For this review, take the finished solid that the model builds, in its own axes (mm). Face numbers are marked on the shaded views. A direction names the side the tool comes from. Coordinates: 2 decimals unless noted, no trailing zeros. Write each loop counter-clockwise with the first axis right and the second up, starting at its lowest first coordinate (ties: lowest second). Pieces come first, ordered by that corner, then holes.
```python
from build123d import *

# Parameters (mm, degrees)
SKETCH1_R           = 17
SKETCH1_R_2         = 13
BOSS_EXTRUDE1_DEPTH = 10
SKETCH2_R           = 30
SKETCH2_R_2         = 13
BOSS_EXTRUDE2_DEPTH = 8
SKETCH6_R           = 17
SKETCH6_R_2         = 8.5
BOSS_EXTRUDE3_DEPTH = 3
SKETCH7_R           = 13
SKETCH7_R_2         = 9.5
BOSS_EXTRUDE4_DEPTH = 9
CUT_EXTRUDE2_START  = -1.8
SKETCH8_R           = 10
CUT_EXTRUDE2_DEPTH  = 1.2


with BuildPart() as part:
    # Sketch1 → Boss-Extrude1 (new body)
    with BuildSketch(Plane.XY):
        Circle(SKETCH1_R)
        Circle(SKETCH1_R_2, mode=Mode.SUBTRACT)
    extrude(amount=BOSS_EXTRUDE1_DEPTH)

    # Sketch2 → Boss-Extrude2 (add)
    with BuildSketch(Plane.XY.offset(10)):
        Circle(SKETCH2_R)
        Circle(SKETCH2_R_2, mode=Mode.SUBTRACT)
    extrude(amount=BOSS_EXTRUDE2_DEPTH)

    # Sketch6 → Boss-Extrude3 (add)
    with BuildSketch(Plane(origin=(0, 0, 0), x_dir=(-1, 0, 0), z_dir=(0, 0, -1))):
        with Locations(Location((0, 0, 0), (0, 0, 180))):
            Circle(SKETCH6_R)
        Circle(SKETCH6_R_2, mode=Mode.SUBTRACT)
    extrude(amount=-BOSS_EXTRUDE3_DEPTH)

    # Sketch7 → Boss-Extrude4 (add)
    with BuildSketch(Plane.XY.offset(3)):
        Circle(SKETCH7_R)
        Circle(SKETCH7_R_2, mode=Mode.SUBTRACT)
    extrude(amount=BOSS_EXTRUDE4_DEPTH)

    # Sketch8 → Cut-Extrude2 (cut)
    with BuildSketch(Plane.XY.offset(12).offset(CUT_EXTRUDE2_START)):
        Circle(SKETCH8_R)
    extrude(amount=-CUT_EXTRUDE2_DEPTH, mode=Mode.SUBTRACT)


solid = part.part
```
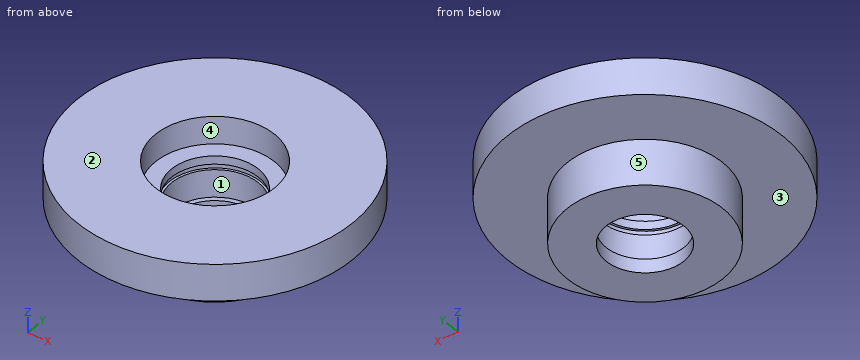
1) Consider section C-C (x = -11). Give the boundary of the cut face in (y, z), then the cut area to 3 significant figures.
2) The part is to be moulded in two halves that separate along Y. For the marked faces 3, 4 and 5, say which applies: pulls with the +Y half, pulls with the -Y half, needs draft (parallel to the pull), parting line crosses it, or undercut.
3) Clearance check with flat-ended pins moving along their axes: P1, Ø10, axis at y = 2, z = 13, coming from the +X side; P2, Ø6, axis at y = 13.5, z = 11.5, coming from the -X side; P3, Ø22, axis at x = 0, y = 0, coming from the +Z side; P4, Ø10, axis at y = -9.5, z = 14, coming from the +X side. State where each tip first meets the part, or that it passes through.
4) Consider section A-A (x = 0). Give the boundary of the cut face in (y, z), then the cut area to 3 significant figures.
5) For L1, parallel to Y at x = 0, z = 15.6; L2, parallel to Y at x = 0, z = 4.45; L3, parallel to Z at x = -24, y = 12, list the stretches that pass through material, from the lowest coordinate up.
6) Tool access review of the marked faces 1 and 2: name each direction out of +Z, -Z, +X, -X, +Y, -Y from which nothing blocks a thin tool from reaching the whole face with its end or side.
7) Consider section D-D (z = 2). Give the boundary of the cut face in (x, y).
Results:
1. outline: (-27.91, 10) - (-12.96, 10) - (-12.96, 0) - (12.96, 0) - (12.96, 10) - (27.91, 10) - (27.91, 18) - (6.93, 18) - (6.93, 12) - (-6.93, 12) - (-6.93, 18) - (-27.91, 18) - close
1. area: 623 mm2
2. face 3: needs draft
2. face 4: undercut
2. face 5: parting line crosses it
3. P1: stops at x = 30
3. P2: stops at x = -28.1
3. P3: stops at z = 12
3. P4: stops at x = 29.66
4. outline: (-30, 10) - (-17, 10) - (-17, 0) - (-8.5, 0) - (-8.5, 3) - (-9.5, 3) - (-9.5, 9) - (-10, 9) - (-10, 10.2) - (-9.5, 10.2) - (-9.5, 12) - (-13, 12) - (-13, 18) - (-30, 18) - close; (8.5, 0) - (17, 0) - (17, 10) - (30, 10) - (30, 18) - (13, 18) - (13, 12) - (9.5, 12) - (9.5, 10.2) - (10, 10.2) - (10, 9) - (9.5, 9) - (9.5, 3) - (8.5, 3) - close
4. area: 441 mm2
5. L1: y = -30 to -13, 13 to 30
5. L2: y = -17 to -9.5, 9.5 to 17
5. L3: z = 10 to 18
6. face 1: +Z
6. face 2: +Z, +X, -X, +Y, -Y
7. outline: circle Ø34 at (0, 0); hole circle Ø17 at (0, 0)
